Autodesk Inventor part; units mm, degrees
ref_plane "YZ Plane" through (0, 0, 0) normal (1, 0, 0) x (0, 1, 0)
ref_plane "XZ Plane" through (0, 0, 0) normal (0, 1, 0) x (-1, 0, 0)
ref_plane "XY Plane" through (0, 0, 0) normal (0, 0, 1) x (1, 0, 0)
sketch "Sketch1" plane through (0, 0, 0) normal (0, 1, 0) x (-1, 0, 0)
  line L0 (0, 0) -> (16.5, 0)
  line L1 (16.5, 0) -> (16.5, -16.5)
  line L2 (16.5, -16.5) -> (0, -16.5)
  line L3 (0, -16.5) -> (0, 0)
  dimension "d0" = 16.5
  dimension "d1" = 16.5
extrude "Extrusion1" add sketch "Sketch1" along normal blind 11
sketch "Sketch2" plane through (0, 0, 0) normal (1, 0, 0) x (0, 0, -1)
  line L0 (0, 0) -> (0, 5)
  line L1 (1, 6) -> (15.5, 6)
  line L2 (16.5, 0) -> (16.5, 11)
  line L3 (16.5, 0) -> (16.5, 5)
  arc A0 (1, 6) -> (0, 5) centre (1, 5) ccw
  arc A1 (16.5, 5) -> (15.5, 6) centre (15.5, 5) ccw
  line L4 (0, 5) -> (0, 6)
  line L5 (1, 7) -> (15.5, 7)
  line L6 (16.5, 5) -> (16.5, 6)
  arc A2 (1, 7) -> (0, 6) centre (1, 6) ccw
  arc A3 (16.5, 6) -> (15.5, 7) centre (15.5, 6) ccw
  line L7 (0, 11) -> (16.5, 11)
  line L8 (16.5, 11) -> (0, 11)
  point P0 (0, 6)
  point P1 (16.5, 6)
  point P2 (0, 7)
  point P3 (16.5, 7)
  dimension "d4" = 6
  dimension "d5" = 1
  dimension "d6" = 2
  dimension "d7" = 1
sketch "Sketch3" plane through (0, 11, 0) normal (0, 1, 0) x (1, 0, 0)
  line L0 (-15.7556, 8.25) -> (-12.0028, 14.75)
  line L1 (-12.0028, 14.75) -> (-4.4972, 14.75)
  line L2 (-4.4972, 14.75) -> (-0.7444, 8.25)
  line L3 (-0.7444, 8.25) -> (-4.4972, 1.75)
  line L4 (-4.4972, 1.75) -> (-12.0028, 1.75)
  line L5 (-12.0028, 1.75) -> (-15.7556, 8.25)
  point P0 (0, 0)
  point P1 (-8.25, 8.25)
  dimension "d8" = 13
extrude "Extrusion2" cut sketch "Sketch3" against normal blind 5
sketch "Sketch4" plane through (0, 6, 0) normal (0, 1, 0) x (1, 0, 0)
  line L0 (-4.4972, 1.75) -> (-12.0028, 1.75)
  line L1 (-12.0028, 14.75) -> (-4.4972, 14.75)
  circle A0 centre (-8.25, 8.25) radius 4
  point P0 (0, 0)
  dimension "d11" = 8
extrude "Extrusion3" cut sketch "Sketch4" against normal blind 20
extrude "Extrusion4" cut sketch "Sketch2" against normal blind 12.5
sketch "Sketch5" plane through (0, 11, 0) normal (0, 1, 0) x (1, 0, 0)
  line L0 (-4.4972, 1.75) -> (-12.0028, 1.75)
  line L1 (-12.0028, 1.75) -> (3.1486, 1.75)
  line L2 (3.1486, 1.75) -> (3.1486, 14.75)
  line L3 (3.1486, 14.75) -> (-12.0028, 14.75)
  line L4 (-12.0028, 14.75) -> (-12.0028, 1.75)
  point P0 (0, 0)
  dimension "d16" = 13
extrude "Extrusion5" cut sketch "Sketch5" against normal up to surface (4 mm away)
sketch "Sketch6" plane through (-16.5, 0, -16.5) normal (-1, 0, 0) x (0, 0, 1)
  line L0 (16.5, 0) -> (0, 0)
  line L1 (16.5, 0) -> (16.5, 11)
  line L2 (0, 11) -> (16.5, 11)
  line L3 (0, 0) -> (0, 11)
extrude "Extrusion6" add sketch "Sketch6" along normal blind 2
sketch "Sketch7" plane through (0, 0, 0) normal (0, -1, 0) x (1, 0, 0)
  circle A0 centre (-8.25, -8.25) radius 4
  line L0 (0, 0) -> (-18.5, 0)
  line L1 (-18.5, -16.5) -> (-18.5, 0)
  line L2 (-18.5, -16.5) -> (0, -16.5)
  line L3 (0, -16.5) -> (0, 0)
extrude "Extrusion7" cut sketch "Sketch7" against normal blind 1
sketch "Sketch8" plane through (0, 11, 0) normal (0, 1, 0) x (1, 0, 0)
  line L0 (0, 1.75) -> (-12.0028, 1.75)
  line L1 (-12.0028, 1.75) -> (-15.7556, 8.25)
  line L2 (-15.7556, 8.25) -> (-12.0028, 14.75)
  line L3 (-12.0028, 14.75) -> (0, 14.75)
  line L4 (0, 14.75) -> (0, 16.5)
  line L5 (0, 16.5) -> (-18.5, 16.5)
  line L6 (-18.5, 0) -> (-18.5, 16.5)
  line L7 (0, 0) -> (-18.5, 0)
  line L8 (0, 0) -> (0, 1.75)
extrude "Extrusion8" add sketch "Sketch8" along normal blind 3
sketch "Sketch10" plane through (0, 7, -1) normal (1, 0, 0) x (0, 0, -1)
  line L0 (15.5, -1) -> (15.5, -2)
  line L1 (15.5, -1) -> (-1, -1)
  line L2 (-1, -1) -> (-1, 0)
  line L3 (0, 1) -> (14.5, 1)
  line L4 (15.5, 0) -> (15.5, -1)
  arc A0 (0, 1) -> (-1, 0) centre (0, 0) ccw
  arc A1 (15.5, 0) -> (14.5, 1) centre (14.5, 0) ccw
  point P0 (-1, -7)
  point P1 (-1, 1)
  point P2 (15.5, 1)
  dimension "d28" = 16.5
  dimension "d29" = 2
  dimension "d30" = 1
extrude "Extrusion9" cut sketch "Sketch10" against normal up to surface (12.5 mm away)
sketch "Sketch11" plane through (0, 5, -16.5) normal (0, 0, -1) x (-1, 0, 0)
  line L0 (18.5, 9) -> (0, 9)
  line L1 (0, 2) -> (0, 9)
  line L2 (18.5, 9) -> (0, 9)
  line L3 (0, 9) -> (0, 2)
  line L4 (0, 2) -> (18.5, 2)
  line L5 (18.5, 2) -> (18.5, 9)
  point P0 (0, -5)
extrude "Extrusion10" add sketch "Sketch11" along normal blind 2
ref_plane "Work Plane1" through (-15.7556, 14, -8.25) normal (0, 0, -1) x (-1, 0, 0)
mirror "Mirror1" about plane through (-15.7556, 14, -8.25) normal (0, 0, -1) of "Extrusion8", "Extrusion10", "Extrusion9", "Extrusion2"
sketch "Sketch12" plane through (-18.5, 0, -16.5) normal (-1, 0, 0) x (0, 0, 1)
  line L0 (18.5, 14) -> (18.5, 7)
  line L1 (18.5, 10.5) -> (-2, 10.5)
  line L2 (-2, 10.5) -> (-2, 3.5)
  line L3 (-2, 3.5) -> (18.5, 3.5)
  line L4 (18.5, 3.5) -> (18.5, 10.5)
  point P0 (16.5, 0)
  point P1 (18.5, 11)
  point P2 (18.5, 9)
extrude "Extrusion11" add sketch "Sketch12" against normal up to surface (6 mm away)
fillet "Fillet3" radius 2 2 edges at (-15.5, 3.5, -18.5) (-15.5, 3.5, 2)
fillet "Fillet4" radius 2 2 edges at (-9.25, 14, -18.5) (-9.25, 14, 2)
fillet "Fillet5" radius 2 2 edges at (-6.25, 7, -16.5) (-6.25, 7, 0)
sketch "Sketch13" plane through (-12.5, 10.5, -2.6112) normal (0, 1, 0) x (1, 0, 0)
  line L0 (-3.2556, 5.6388) -> (0, 11.2776)
  line L1 (0, 0) -> (-3.2556, 5.6388)
  line L2 (0, 0) -> (0, 11.2776)
  point P0 (12.5, -2.6112)
extrude "Extrusion12" cut sketch "Sketch13" against normal blind 3
sketch "Sketch14" plane through (-12.5, 0, 0) normal (1, 0, 0) x (0, 0, -1)
  line L0 (13.8888, 8) -> (13.8888, 7.5)
  line L1 (13.8888, 7.5) -> (2.6112, 7.5)
  line L2 (2.6112, 7.5) -> (2.6112, 8)
  line L3 (1, 8) -> (2.6112, 8)
  arc A0 (1, 8) -> (0.2546, 7.6667) centre (1, 7) ccw
  arc A1 (-1.2361, 7) -> (0.2546, 7.6667) centre (-1.2361, 9) ccw
  line L4 (-2, 7) -> (-1.2361, 7)
  line L5 (-2, 5.5) -> (-2, 7)
  arc A2 (-2, 5.5) -> (0, 3.5) centre (0, 5.5) ccw
  line L6 (0, 5) -> (0, 3.5)
  arc A3 (1, 6) -> (0, 5) centre (1, 5) ccw
  line L7 (15.5, 6) -> (1, 6)
  arc A4 (16.5, 5) -> (15.5, 6) centre (15.5, 5) ccw
  line L8 (16.5, 3.5) -> (16.5, 5)
  arc A5 (16.5, 3.5) -> (18.5, 5.5) centre (16.5, 5.5) ccw
  line L9 (18.5, 7) -> (18.5, 5.5)
  line L10 (17.7361, 7) -> (18.5, 7)
  arc A6 (16.2454, 7.6667) -> (17.7361, 7) centre (17.7361, 9) ccw
  arc A7 (16.2454, 7.6667) -> (15.5, 8) centre (15.5, 7) ccw
  line L11 (13.8888, 8) -> (15.5, 8)
  line L12 (13.8888, 8) -> (2.6112, 8)
  line L13 (2.6112, 8) -> (2.6112, 7.5)
  line L14 (2.6112, 7.5) -> (13.8888, 7.5)
  line L15 (13.8888, 7.5) -> (13.8888, 8)
  point P0 (0, 0)
extrude "Extrusion13" cut sketch "Sketch14" against normal blind 2
sketch "Sketch15" plane through (0, 14, 0) normal (0, 1, 0) x (1, 0, 0)
  line L0 (0, 0) -> (-18.5, 0)
  line L1 (0, 1.75) -> (0, 0)
  line L2 (0, 1.75) -> (-12.0028, 1.75)
  line L3 (-12.0028, 1.75) -> (-15.7556, 8.25)
  line L4 (-15.7556, 8.25) -> (-12.0028, 14.75)
  line L5 (-12.0028, 14.75) -> (0, 14.75)
  line L6 (0, 14.75) -> (0, 16.5)
  line L7 (-18.5, 16.5) -> (0, 16.5)
  line L8 (-18.5, 0) -> (-18.5, 16.5)
  line L9 (-11.7141, 14.25) -> (-15.1782, 8.25)
  line L10 (-15.1782, 8.25) -> (-11.7141, 2.25)
  line L11 (-11.7141, 2.25) -> (0, 2.25)
  line L12 (0, -0.5) -> (-19, -0.5)
  line L13 (-19, -0.5) -> (-19, 17)
  line L14 (-19, 17) -> (0, 17)
  line L15 (0, 14.25) -> (-11.7141, 14.25)
  line L16 (0, 14.75) -> (0, 14.25)
  line L17 (0, 2.25) -> (0, 1.75)
  line L18 (0.5, 2.25) -> (0.5, 1.75)
  line L19 (0.5, 14.75) -> (0.5, 14.25)
  point P0 (0, 0)
  dimension "d45" = 0.5
extrude "Extrusion14" add sketch "Sketch15" against normal blind 1 contours L2 L3 L4 L5 L16 L15 L9 L10 L11 L17
move or copy body "Move Body1" bodies to move or copy 1 copy no translate (0, 2, 0)
properties part number "nut holder"
The model under review builds one solid part; all positions refer to its coordinate system, in mm. A direction names the side the tool comes from. Give positions to 0.01 mm unless a question says otherwise; leave off trailing zeros. Write each loop counter-clockwise with the first axis right and the second up, starting at its lowest first coordinate (ties: lowest second). Pieces come first, ordered by that corner, then holes. Notation, with made-up numbers: M 40.5,44 L 65.5,44 A7 cw 65.5,55 Z; hole C 32,3 d9. An arc over 180 degrees is marked long. Write each question's results on one line, items separated by ' | '. Start each with the question number.
1. For faces 1 (the flat face through (-5.9, 15.5, -2.25)), 2 (the cylindrical face through (-13.49, 9.17, 0.43)), 3 (the cylindrical face through (-7.148, 7.699, -16.215)), list the 3-axis set-ups (+Z, -Z, +X, -X, +Y, -Y) from which the entire face can be reached by the end or side of a thin tool; tool diameter is ignored.
2. For probe 1 along X at (y, z) = (4.55, -8.25); probe 2 along Z at (x, y) = (-8.25, 5.95); probe 3 along Y at (x, z) = (-14, -15.25), list the stretches that pass through material, from the lowest coordinate up. Write a range as [from, to].
3. Insertion check: pin 1 Ø0.6 at (x, z) = (-8.5, 1.5) entering from -Y; pin 2 Ø4 at (x, z) = (-9.5, -5.5) entering from +Y; pin 3 Ø4.5 at (x, y) = (-9, 5.5) entering from -Z. Each pin has a flat end and moves straight along its axis. Give the tip position at first contact, or say it passes through.
4. We need section C-C (y = 11). Write out the cut boundary in (x, z), and give its area (3 significant figures).
5. Mouldability with a two-part tool opening along Z and no side actions: class faces 4 (the flat face through (-6, 12, -14.75)), 5 (the flat face through (-16, 16, -8)), 6 (the cylindrical face through (-9.12, 15.43, 1.4)) as released by +Z, released by -Z, zero draft, split by the parting line, or undercut.
6. We need section D-D (x = -8.25). Count the separate pieces of the cut face and the enclosed holes in it, and give its area (3 significant figures).
7. We need section A-A (z = -9.25). Write out the cut boundary in (x, y), and give its area (3 significant figures).
Results found:
1) face 1: +X, +Y | face 2: +X | face 3: -Z, +X
2) probe 1: x = [-18.5, -12.25], [-4.25, 0] | probe 2: z = [-16.5, -12.25], [-4.25, 0] | probe 3: y = [3, 8], [10, 16]
3) pin 1: stops at y = 9 | pin 2: stops at y = 8 | pin 3: stops at z = -16.5
4) outline: M -18.5,-18.5 L 0,-18.5 L 0,-14.75 L -12,-14.75 L -12.5,-13.89 L -15.76,-8.25 L -12.5,-2.61 L -12,-1.75 L 0,-1.75 L 0,2 L -18.5,2 Z | area: 199 mm^2
5) face 4: undercut | face 5: zero draft | face 6: released by +Z
6) separate pieces: 4 | enclosed holes: 0 | area: 90.4 mm^2
7) outline: M -18.5,3 L -12.12,3 L -12.12,8 L -14.5,8 L -14.5,9.5 L -15.18,9.5 L -15.18,15 L -14.6,15 L -14.6,16 L -18.5,16 Z; M -4.38,3 L 0,3 L 0,8 L -4.38,8 Z | area: 81.9 mm^2
